CAD build for the part. Positions are in the model's coordinates, mm. A direction names the side the tool comes from. Round coordinates to 2 decimals unless told otherwise and drop trailing zeros. Loops run counter-clockwise (first coordinate to the right, second up) from the corner with the lowest first, then second, coordinate; pieces in that order, holes last. Notation, with made-up numbers: (-37.5, 10.25) - (13.5, 10.25) arc R15 ccw to (13.5, 36.25) - close; hole circle Ø8 at (19, 50.25). An arc over 180 degrees is marked (long way). Use one line per item in the form item = value.
from build123d import *

# Parameters (mm, degrees)
F0_W     = 81.626944
F0_H     = 51.38012
F1_DEPTH = 6.35
F2_W     = 92.995196
F2_H     = 57.772774
F2_W_2   = 81.00345
F2_H_2   = 50.874696
F3_DEPTH = 12.7
F4_W     = 78.571246
F4_H     = 46.661102
F5_DEPTH = 25.4
F6_W     = 53.555076
F6_H     = 27.672314
F7_DEPTH = 12.7


with BuildPart() as f1:
    # F0 (on Front) → F1 (new body)
    with BuildSketch(Plane.XZ):
        Rectangle(F0_W, F0_H)
    extrude(amount=F1_DEPTH)

    # F2 (on Front) → F3 (join)
    with BuildSketch(Plane.XZ):
        Rectangle(F2_W, F2_H)
        Rectangle(F2_W_2, F2_H_2, mode=Mode.SUBTRACT)
    extrude(amount=F3_DEPTH)

    # F4 (on face) → F5 (join)
    with BuildSketch(Plane(origin=(0, 0, 0), x_dir=(-1, 0, 0), z_dir=(0, 1, 0))):
        Rectangle(F4_W, F4_H)
    extrude(amount=F5_DEPTH)

    # F6 (on face) → F7 (join)
    with BuildSketch(Plane(origin=(0, 25.4, 0), x_dir=(-1, 0, 0), z_dir=(0, 1, 0))):
        with Locations((0, -4.375952)):
            Rectangle(F6_W, F6_H)
    extrude(amount=F7_DEPTH)


solid = f1.part
1) Slice it at D-D (y = 22). Write the cut outline in (x, z).
Report:
outline = (-39.29, -23.33) - (39.29, -23.33) - (39.29, 23.33) - (-39.29, 23.33) - close
2) Slice it at A-A (x = -19). Write the cut outline in (y, z), plus the area to 3 significant figures.
Report:
outline = (-12.7, -28.89) - (0, -28.89) - (0, -23.33) - (25.4, -23.33) - (25.4, -18.21) - (38.1, -18.21) - (38.1, 9.46) - (25.4, 9.46) - (25.4, 23.33) - (0, 23.33) - (0, 28.89) - (-12.7, 28.89) - (-12.7, 25.44) - (-6.35, 25.44) - (-6.35, -25.44) - (-12.7, -25.44) - close
area = 1,950 mm^2
3) Tool access for faces 1 (the flat face through (-26.778, 32, -5)), 2 (the flat face through (26.778, 32, -5)), 3 (the flat face through (1, 13, -23.331)), 4 (the flat face through (-1, -6.35, 0)): list every direction of +Z, -Z, +X, -X, +Y, -Y with a clear straight run to the whole face (end or side of a thin tool).
Report:
face_1 = +Z, -Z, -X, +Y
face_2 = +Z, -Z, +X, +Y
face_3 = -Z, +X, -X, +Y
face_4 = -Y
4) Slice it at B-B (z = 11.5). Write the cut outline in (x, y), plus the area to 3 significant figures.
Report:
outline = (-46.5, -12.7) - (-40.5, -12.7) - (-40.5, -6.35) - (40.5, -6.35) - (40.5, -12.7) - (46.5, -12.7) - (46.5, 0) - (39.29, 0) - (39.29, 25.4) - (-39.29, 25.4) - (-39.29, 0) - (-46.5, 0) - close
area = 2,660 mm^2
5) Slice it at C-C (x = -35). Write the cut outline in (y, z).
Report:
outline = (-12.7, -28.89) - (0, -28.89) - (0, -23.33) - (25.4, -23.33) - (25.4, 23.33) - (0, 23.33) - (0, 28.89) - (-12.7, 28.89) - (-12.7, 25.44) - (-6.35, 25.44) - (-6.35, -25.44) - (-12.7, -25.44) - close
6) Drill centre lines: probe 1 along Z at (x, y) = (9, -9.5); probe 2 along X at (y, z) = (-8, 16.5); probe 3 along Y at (x, z) = (-8, -19.5). Where is each one in solid material? Low to high.
Report:
probe_1 = -28.89 to -25.44, 25.44 to 28.89
probe_2 = -46.5 to -40.5, 40.5 to 46.5
probe_3 = -6.35 to 25.4
7) Two-plate mould, pull along X, no slides. Class faces 5 (the flat face through (-46.498, -6, 0)), 6 (the flat face through (1, 13, 23.331)), 7 (the flat face through (-1, -9, -25.437)): +X half, -X half, draft (parallel to the pull), parting line (faces both ways), or undercut.
Report:
face_5 = -X half
face_6 = draft
face_7 = undercut
8) Flat gauge pins, fed straight in: pin 1 (10 mm diameter, centred on x = -5.5, y = 35, fed in from +Z); pin 2 (4 mm diameter, centred on y = 32.5, z = -2.5, fed in from -X); pin 3 (6 mm diameter, centred on x = 15, z = 6, fed in from -Y). Where does each tip first touch, or does it go through?
Report:
pin_1 = 9.46
pin_2 = -26.78
pin_3 = -6.35
